Job drawing, mm, ordinate dimensions from the low corner. One solid piece. Coordinates: 2 decimals unless noted, no trailing zeros. Write each loop counter-clockwise with the first axis right and the second up, starting at its lowest first coordinate (ties: lowest second). Pieces come first, ordered by that corner, then holes.
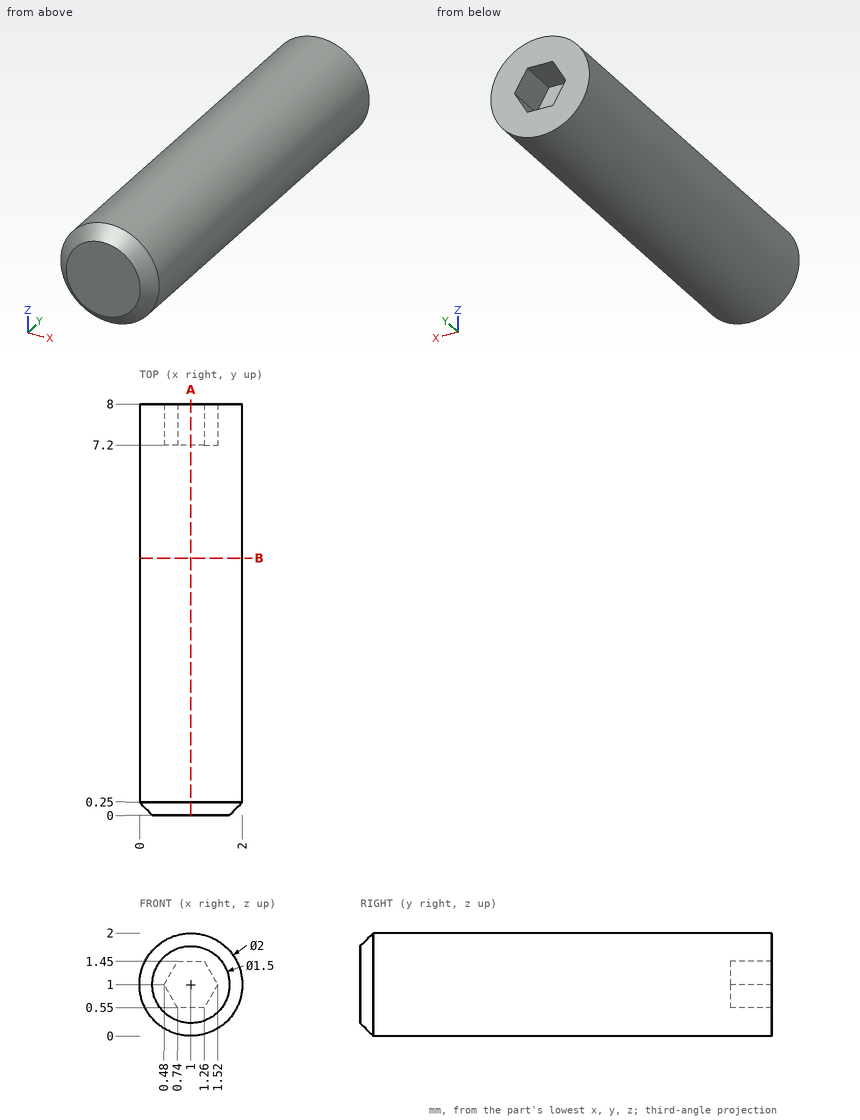
1. Saw through at A-A on x = 1. List the corners of the cut face in (y, z), plus the area to 3 significant figures.
Computed values:
outline: (0, 0.25) - (0.25, 0) - (8, 0) - (8, 0.55) - (7.2, 0.55) - (7.2, 1.45) - (8, 1.45) - (8, 2) - (0.25, 2) - (0, 1.75) - close
area: 15.2 mm2
2. Probe line 1 along Y through (x, z) = (1, 1.1); line 2 along Z through (x, y) = (1.3, 1.5) (1 decimal); line 3 along Z through (x, y) = (1.4, 3.5). List the from-to ranges inside material, lowest first.
Computed values:
line 1: y = 0 to 7.2
line 2: z = 0 to 2
line 3: z = 0.08 to 1.92
3. Flat gauge pin, fed straight in: pin 1 (1 mm diameter, centred on x = 1, z = 0, fed in from -Y). Where does the tip first touch, or does it go through?
Computed values:
pin 1: stops at y = 0
4. Saw through at B-B on y = 5. List the corners of the cut face in (x, z).
Computed values:
outline: circle Ø2 at (1, 1)
